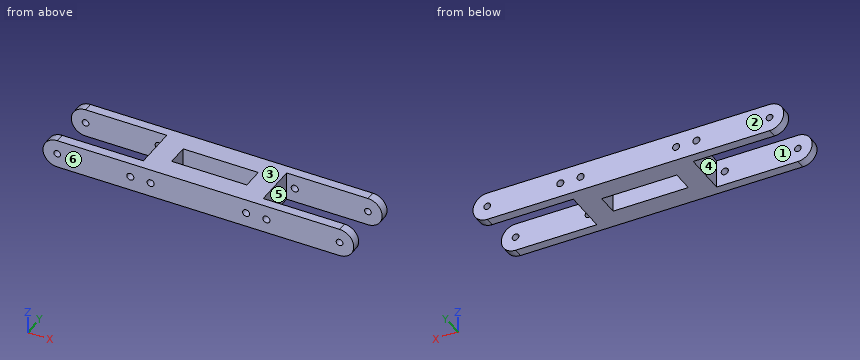
```python
from build123d import *

# Parameters (mm, degrees)
SKETCH_1_R          = 1.65
SKETCH_1_R_2        = 1.75
EXTRUDE_1_DEPTH     = 30.5
CUT_EXTRUDE_1_DEPTH = 62.051208014
SKETCH_3_W          = 20
SKETCH_3_H          = 10.5
CUT_EXTRUDE_2_DEPTH = 62.051208014
SKETCH_4_W          = 18.5
SKETCH_4_H          = 10
EXTRUDE_2_DEPTH     = 14
SKETCH_5_W          = 11
SKETCH_5_H          = 10.5
EXTRUDE_3_DEPTH     = 14


with BuildPart() as part:
    # Sketch 1 → Extrude 1 (new body)
    with BuildSketch(Plane(origin=(0, 0, 0), x_dir=(1, 0, 0), z_dir=(0, 1, 0))):
        with BuildLine():
            Line((0, 7), (51, 7))
            Line((51, 7), (51, -7))
            Line((51, -7), (0, -7))
            ThreePointArc((0, -7), (-7, 0), (0, 7))
        make_face()
        with Locations(Location((0, 0, 0), (0, 0, 90))):
            Circle(SKETCH_1_R, mode=Mode.SUBTRACT)
        with Locations(Location((46, 0, 0), (0, 0, 90))):
            Circle(SKETCH_1_R_2, mode=Mode.SUBTRACT)
        with Locations(Location((36, 0, 0), (0, 0, 90))):
            Circle(SKETCH_1_R_2, mode=Mode.SUBTRACT)
    extrude(amount=EXTRUDE_1_DEPTH)

    # Sketch 2 → Cut-Extrude 1 (cut, through all)
    with BuildSketch(Plane.XY.offset(7)):
        Polygon((0, 26), (-7, 26), (-7, 4.5), (0, 4.5), (40, 4.5), (40, 26), align=None)
    extrude(amount=-CUT_EXTRUDE_1_DEPTH, mode=Mode.SUBTRACT)

    # Sketch 3 → Cut-Extrude 2 (cut, through all)
    with BuildSketch(Plane.XY.offset(7)):
        with Locations((41, 15.25)):
            Rectangle(SKETCH_3_W, SKETCH_3_H)
    extrude(amount=-CUT_EXTRUDE_2_DEPTH, mode=Mode.SUBTRACT)


with BuildPart() as cut_extrude_2_piece_1:
    # of the separate pieces the step leaves, piece 1, a body of its own (cut_extrude_2_pieces)
    add(part.part.solids().sort_by_distance((51, 20.5, -7))[0])


with BuildPart() as cut_extrude_2_piece_2:
    # of the separate pieces the step leaves, piece 2, a body of its own (cut_extrude_2_pieces)
    add(part.part.solids().sort_by_distance((0, 0, -7))[0])

    # Sketch 4 → Extrude 2 (add)
    with BuildSketch(Plane.XY.offset(7)):
        with Locations((60.25, 25.5)):
            Rectangle(SKETCH_4_W, SKETCH_4_H)
        with Locations((60.25, 5)):
            Rectangle(SKETCH_4_W, SKETCH_4_H)
    extrude(amount=-EXTRUDE_2_DEPTH)


with BuildPart() as extrude_2_piece_1:
    # of the separate pieces the step leaves, piece 1, a body of its own (extrude_2_pieces)
    add(cut_extrude_2_piece_2.part.solids().sort_by_distance((0, 0, -7))[0])

    # Mirror 1: Extrude 2 piece 1 across plane


with BuildPart() as extrude_2_piece_2:
    # of the separate pieces the step leaves, piece 2, a body of its own (extrude_2_pieces)
    add(cut_extrude_2_piece_2.part.solids().sort_by_distance((51, 30.5, 7))[0])


with BuildPart() as extrude_2_piece_1_1:
    add(extrude_2_piece_1.part)
    add(extrude_2_piece_1.part.mirror(Plane(origin=(69.5, 10, -7), x_dir=(0, 0, 1), z_dir=(1, 0, 0))))


with BuildPart() as body_4:
    # Mirror 2: mirrored copy
    add(extrude_2_piece_2.part.mirror(Plane(origin=(69.5, 30.5, -7), x_dir=(0, 0, 1), z_dir=(1, 0, 0))))


with BuildPart() as body_5:
    # Mirror 2 2: mirrored copy
    add(cut_extrude_2_piece_1.part.mirror(Plane(origin=(69.5, 30.5, -7), x_dir=(0, 0, 1), z_dir=(1, 0, 0))))


with BuildPart() as cut_extrude_2_piece_1_1:
    add(cut_extrude_2_piece_1.part)

    add(extrude_2_piece_1_1.part)  # Extrude 3 merges Extrude 2 piece 1

    add(extrude_2_piece_2.part)  # Extrude 3 merges Extrude 2 piece 2

    add(body_4.part)  # Extrude 3 merges body 4

    add(body_5.part)  # Extrude 3 merges body 5
    # Sketch 5 → Extrude 3 (add)
    with BuildSketch(Plane(origin=(0, 0, -7), x_dir=(-1, 0, 0), z_dir=(0, 0, -1))):
        with Locations((-93.5, 15.25)):
            Rectangle(SKETCH_5_W, SKETCH_5_H)
        with Locations((-45.5, 15.25)):
            Rectangle(SKETCH_5_W, SKETCH_5_H)
    extrude(amount=-EXTRUDE_3_DEPTH)


solid = cut_extrude_2_piece_1_1.part
```
For this review, take the finished solid that the model builds, in its own axes (mm). Face numbers are marked on the shaded views. A direction names the side the tool comes from. Coordinates: 2 decimals unless noted, no trailing zeros. Order: outer loops, then holes, each group sorted by start corner. A loop starts at its lowest first (then second) coordinate and runs counter-clockwise, first axis right, second up. Notation, with made-up numbers: (48.5, -31.75) - (75.5, -31.75) arc R22 cw to (75.5, -1.75) - close; hole circle Ø1 at (14.5, 26). An arc over 180 degrees is marked (long way). Answer as a JSON object with one key per item and string values. Group by question number.
1. The part is to be moulded in two halves that separate along Y. For the marked faces 1, 2 and 3, say which applies: pulls with the +Y half, pulls with the -Y half, needs draft (parallel to the pull), parting line crosses it, or undercut.
2. We need section D-D on y = 12. State the section outline as (x, z) points.
3. For the marked faces 4, 5 and 6, list the 3-axis set-ups (+Z, -Z, +X, -X, +Y, -Y) from which the entire face can be reached by the end or side of a thin tool; tool diameter is ignored.
4. We need section A-A on x = 58. State the section outline as (y, z) points, then the cut area to 3 significant figures.
5. Clearance check with flat-ended pins moving along their axes: P1, Ø3, axis at y = 11, z = -3.5, coming from the +X side; P2, Ø5, axis at y = 13.5, z = -3, coming from the -X side; P3, Ø1, axis at x = 46.5, z = 1, coming from the -Y side. State where each tip first meets the part, or that it passes through.
6. We need section C-C on y = 2. State the section outline as (x, z) points, then the cut area to 3 significant figures.
7. For probe 1 along X at (y, z) = (25.5, -0.25); probe 2 along Y at (x, z) = (4, -5.25); probe 3 along X at (y, z) = (24.5, 1.25), list the stretches that pass through material, from the lowest coordinate up.
8. We need section B-B on x = 36. State the section outline as (y, z) points, then the cut area to 3 significant figures.
Final values:
{
 "1": {"face 1": "undercut", "face 2": "pulls with the +Y half", "face 3": "needs draft"},
 "2": {"outline": "(40, -7) - (51, -7) - (51, 7) - (40, 7) - close; (88, -7) - (99, -7) - (99, 7) - (88, 7) - close"},
 "3": {"face 4": "+Z, -Z, -X", "face 5": "+Z, -Z, +X", "face 6": "+Z, -Z, +X, -X, -Y"},
 "4": {"outline": "(0, -7) - (10, -7) - (10, 7) - (0, 7) - close; (20.5, -7) - (30.5, -7) - (30.5, 7) - (20.5, 7) - close", "area": "280 mm²"},
 "5": {"P1": "x = 99", "P2": "x = 40", "P3": "y = 10"},
 "6": {"outline": "(0, -7) - (139, -7) arc R7 ccw to (139, 7) - (0, 7) arc R7 ccw to start; hole circle Ø3.3 at (0, 0); hole circle Ø3.5 at (36, 0); hole circle Ø3.5 at (46, 0); hole circle Ø3.5 at (93, 0); hole circle Ø3.5 at (103, 0); hole circle Ø3.3 at (139, 0)", "area": "2,040 mm²"},
 "7": {"probe 1": "40 to 44.27, 47.73 to 91.27, 94.73 to 99", "probe 2": "0 to 4.5, 26 to 30.5", "probe 3": "40 to 44.78, 47.22 to 91.78, 94.22 to 99"},
 "8": {"outline": "(0, -7) - (4.5, -7) - (4.5, -1.75) - (0, -1.75) - close; (0, 1.75) - (4.5, 1.75) - (4.5, 7) - (0, 7) - close; (26, -7) - (30.5, -7) - (30.5, -1.75) - (26, -1.75) - close; (26, 1.75) - (30.5, 1.75) - (30.5, 7) - (26, 7) - close", "area": "94.5 mm²"}
}
